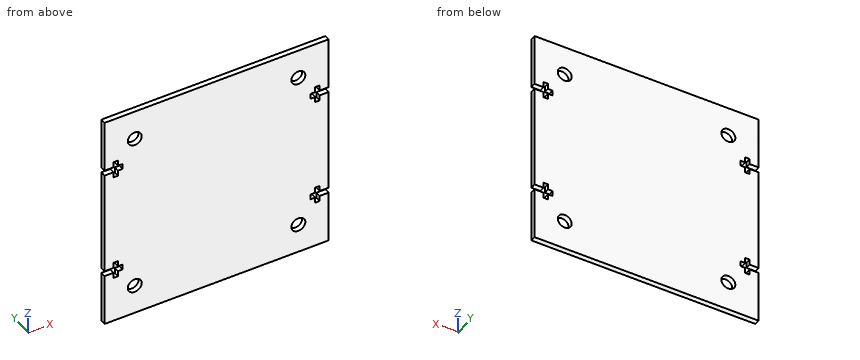
from build123d import *

# Parameters (mm, degrees)
BOSS_EXTRUDE1_DEPTH = 2.9718
SKETCH3_R           = 3.96875
CUT_EXTRUDE1_DEPTH  = 2.9718


with BuildPart() as part:
    # Sketch2 → Boss-Extrude1 (new body)
    with BuildSketch(Plane(origin=(0, 0, 0), x_dir=(1, 0, 0), z_dir=(0, 1, 0))):
        Polygon((0, 30.2006), (0, 0), (127, 0), (127, 30.2006), (121.92, 30.2006), (121.92, 26.9875), (119.38, 26.9875), (119.38, 30.2006), (116.84, 30.2006), (116.84, 33.2994), (119.38, 33.2994), (119.38, 36.5125), (121.92, 36.5125), (121.92, 33.2994), (127, 33.2994), (127, 63.5), (127, 93.7006), (121.92, 93.7006), (121.92, 90.4875), (119.38, 90.4875), (119.38, 93.7006), (116.84, 93.7006), (116.84, 96.7994), (119.38, 96.7994), (119.38, 100.0125), (121.92, 100.0125), (121.92, 96.7994), (127, 96.7994), (127, 127), (0, 127), (0, 96.7994), (5.08, 96.7994), (5.08, 100.0125), (7.62, 100.0125), (7.62, 96.7994), (10.16, 96.7994), (10.16, 93.7006), (7.62, 93.7006), (7.62, 90.4875), (5.08, 90.4875), (5.08, 93.7006), (0, 93.7006), (0, 63.5), (0, 33.2994), (5.08, 33.2994), (5.08, 36.5125), (7.62, 36.5125), (7.62, 33.2994), (10.16, 33.2994), (10.16, 30.2006), (7.62, 30.2006), (7.62, 26.9875), (5.08, 26.9875), (5.08, 30.2006), align=None)
    extrude(amount=BOSS_EXTRUDE1_DEPTH)

    # Sketch3 → Cut-Extrude1 (cut)
    with BuildSketch(Plane(origin=(0, 2.9718, 0), x_dir=(1, 0, 0), z_dir=(0, 1, 0))):
        with Locations(Location((17.145, 109.855, 0), (0, 0, 270))):
            Circle(SKETCH3_R)
        with Locations(Location((109.855, 109.855, 0), (0, 0, 270))):
            Circle(SKETCH3_R)
        with Locations(Location((109.855, 17.145, 0), (0, 0, 270))):
            Circle(SKETCH3_R)
        with Locations(Location((17.145, 17.145, 0), (0, 0, 270))):
            Circle(SKETCH3_R)
    extrude(amount=-CUT_EXTRUDE1_DEPTH, mode=Mode.SUBTRACT)


solid = part.part
Model file for the job. Use its own axes, mm. Give positions to 0.01 mm unless a question says otherwise; leave off trailing zeros. Loops run counter-clockwise (first coordinate to the right, second up) from the corner with the lowest first, then second, coordinate; pieces in that order, holes last.
Item 1: Slice it at A-A (z = -92). Write the cut outline in (x, y), plus the area to 3 significant figures.
Check values:
outline: (0, 0) - (5.08, 0) - (5.08, 2.97) - (0, 2.97) - close; (7.62, 0) - (119.38, 0) - (119.38, 2.97) - (7.62, 2.97) - close; (121.92, 0) - (127, 0) - (127, 2.97) - (121.92, 2.97) - close
area: 362 mm2
Item 2: Slice it at B-B (z = -15). Write the cut outline in (x, y).
Check values:
outline: (0, 0) - (13.81, 0) - (13.81, 2.97) - (0, 2.97) - close; (20.48, 0) - (106.52, 0) - (106.52, 2.97) - (20.48, 2.97) - close; (113.19, 0) - (127, 0) - (127, 2.97) - (113.19, 2.97) - close
Item 3: Drill centre lines: line 1 along Z through (x, y) = (117.5, 1.3); line 2 along Z through (x, y) = (6, 0.65); line 3 along X through (y, z) = (0.35, -29). Where is each one in solid material? Low to high.
Check values:
line 1: z = -127 to -96.8, -93.7 to -33.3, -30.2 to 0
line 2: z = -127 to -100.01, -90.49 to -36.51, -26.99 to 0
line 3: x = 0 to 5.08, 7.62 to 119.38, 121.92 to 127
Item 4: Slice it at C-C (y = 2.05). Give the number of separate pieces and of enclosed holes in the cut face, plus the area to 3 significant figures.
Check values:
separate pieces: 1
enclosed holes: 4
area: 15,700 mm2
